```python
from build123d import *

# Parameters (mm, degrees)
SKETCH1_W                                = 10
SKETCH1_H                                = 31
BOSS_EXTRUDE1_DEPTH                      = 10
SKETCH2_W                                = 3
SKETCH2_H                                = 8.5
CUT_EXTRUDE1_DEPTH                       = 10
CBORE_FOR_M2_PAN_HEAD_SCREW1_D           = 2.4
CBORE_FOR_M2_PAN_HEAD_SCREW1_DEPTH       = 10
CBORE_FOR_M2_PAN_HEAD_SCREW1_CBORE_D     = 5
CBORE_FOR_M2_PAN_HEAD_SCREW1_CBORE_DEPTH = 1.6
CBORE_FOR_M2_PAN_HEAD_SCREW1_TIP         = 0.721032743


with BuildPart() as part:
    # Sketch1 → Boss-Extrude1 (new body)
    with BuildSketch(Plane.XY):
        with Locations((5, 15.5)):
            Rectangle(SKETCH1_W, SKETCH1_H)
    extrude(amount=BOSS_EXTRUDE1_DEPTH)

    # Sketch2 → Cut-Extrude1 (cut)
    with BuildSketch(Plane.XY.offset(10)):
        with Locations((8.5, 26.75)):
            Rectangle(SKETCH2_W, SKETCH2_H)
    extrude(amount=-CUT_EXTRUDE1_DEPTH, mode=Mode.SUBTRACT)

    # CBORE for M2 Pan Head Screw1
    with Locations(Plane.XY.offset(10)):
        with Locations((5, 14), (5, 6)):
            CounterBoreHole(CBORE_FOR_M2_PAN_HEAD_SCREW1_D / 2, CBORE_FOR_M2_PAN_HEAD_SCREW1_CBORE_D / 2, CBORE_FOR_M2_PAN_HEAD_SCREW1_CBORE_DEPTH, depth=CBORE_FOR_M2_PAN_HEAD_SCREW1_DEPTH)
            with Locations((0, 0, -(CBORE_FOR_M2_PAN_HEAD_SCREW1_DEPTH + CBORE_FOR_M2_PAN_HEAD_SCREW1_TIP / 2))):  # 118° drill point
                Cone(0, CBORE_FOR_M2_PAN_HEAD_SCREW1_D / 2, CBORE_FOR_M2_PAN_HEAD_SCREW1_TIP, mode=Mode.SUBTRACT)


solid = part.part
```
Could you check a few things on this model? Use its own coordinates, in mm. A direction names the side the tool comes from. Round coordinates to 2 decimals unless told otherwise and drop trailing zeros. Loops run counter-clockwise (first coordinate to the right, second up) from the corner with the lowest first, then second, coordinate; pieces in that order, holes last.
Q1. I want a section at D-D (x = 3.25). Write out the boundary of the cut face in (y, z).
Q2. I want a section at B-B (y = 14). Write out the boundary of the cut face in (x, z).
Q3. Please list where these lines run through material, in increasing order: L1, parallel to Y at x = 5, z = 5.25; L2, parallel to Y at x = 5, z = 8.85; L3, parallel to Y at x = 9.25, z = 2.5.
Q4. On a 3-axis mill with a long thin cutter (end or side, diameter ignored), from which of +Z, -Z, +X, -X, +Y, -Y can I reach the whole of each face in a straight line? I mean faces 1 (the flat face through (10, 11, 5)), 2 (the cylindrical face through (7.385, 6.751, 9.211)). Say none if no direction works.
Q5. For P1, Ø2, axis at x = 3.5, z = 9, coming from the -Y side; P2, Ø1.4, axis at x = 5, y = 6, coming from the +Z side; P3, Ø3, axis at x = 5, y = 14, coming from the +Z side, each with a flat end and sliding along its axis, tell me the tip position at first contact or that it passes through.
Q6. Thinking about a two-plate mould opening in X: for faces 3 (the flat face through (7, 27, 5)), 4 (the flat face through (8, 22.5, 5)), 5 (the cylindrical face through (6.2, 6.05, 4.14)), 6 (the flat face through (6, 7, 8.4)), which applies, pulls with the +X half, pulls with the -X half, needs draft (parallel to the pull), parting line crosses it, or undercut?
Q7. I want a section at A-A (x = 5). Write out the boundary of the cut face in (y, z), and give its area (3 significant figures).
Q8. I want a section at C-C (z = 2). Write out the boundary of the cut face in (x, y), and give its area (3 significant figures).
Answer below:
1. outline: (0, 0) - (31, 0) - (31, 10) - (15.79, 10) - (15.79, 8.4) - (12.21, 8.4) - (12.21, 10) - (7.79, 10) - (7.79, 8.4) - (4.21, 8.4) - (4.21, 10) - (0, 10) - close
2. outline: (0, 0) - (3.8, 0) - (3.8, 8.4) - (2.5, 8.4) - (2.5, 10) - (0, 10) - close; (6.2, 0) - (10, 0) - (10, 10) - (7.5, 10) - (7.5, 8.4) - (6.2, 8.4) - close
3. L1: y = 0 to 4.8, 7.2 to 12.8, 15.2 to 31
3. L2: y = 0 to 3.5, 8.5 to 11.5, 16.5 to 31
3. L3: y = 0 to 22.5
4. face 1: +Z, -Z, +X, +Y, -Y
4. face 2: +Z
5. P1: stops at y = 0
5. P2: passes through
5. P3: stops at z = 8.4
6. face 3: pulls with the +X half
6. face 4: needs draft
6. face 5: undercut
6. face 6: undercut
7. outline: (0, 0) - (4.8, 0) - (4.8, 8.4) - (3.5, 8.4) - (3.5, 10) - (0, 10) - close; (7.2, 0) - (12.8, 0) - (12.8, 8.4) - (11.5, 8.4) - (11.5, 10) - (8.5, 10) - (8.5, 8.4) - (7.2, 8.4) - close; (15.2, 0) - (31, 0) - (31, 10) - (16.5, 10) - (16.5, 8.4) - (15.2, 8.4) - close
7. area: 254 mm2
8. outline: (0, 0) - (10, 0) - (10, 22.5) - (7, 22.5) - (7, 31) - (0, 31) - close; hole circle Ø2.4 at (5, 6); hole circle Ø2.4 at (5, 14)
8. area: 275 mm2
